from build123d import *

# Parameters (mm, degrees)
F0_W     = 60
F0_H     = 60
F0_R     = 1.25
F0_W_2   = 40.8
F0_H_2   = 40.8
F1_DEPTH = 7
F0_W_3   = 35
F0_H_3   = 35
F2_DEPTH = 2
F3_SIZE  = 1
F4_SIZE  = 1


with BuildPart() as f1:
    # F0 (on Front) → F1 (new body)
    with BuildSketch(Plane.XZ):
        Rectangle(F0_W, F0_H)
        with Locations((-25, -25)):
            Circle(F0_R, mode=Mode.SUBTRACT)
        with Locations((25, -25)):
            Circle(F0_R, mode=Mode.SUBTRACT)
        with Locations((-25, 25)):
            Circle(F0_R, mode=Mode.SUBTRACT)
        Rectangle(F0_W_2, F0_H_2, mode=Mode.SUBTRACT)
        with Locations((25, 25)):
            Circle(F0_R, mode=Mode.SUBTRACT)
    extrude(amount=F1_DEPTH)

    # F0 (on Front) → F2 (join)
    with BuildSketch(Plane.XZ):
        Rectangle(F0_W_2, F0_H_2)
        Rectangle(F0_W_3, F0_H_3, mode=Mode.SUBTRACT)
    extrude(amount=F2_DEPTH)

    # F3
    f3_edges = [f1.edges().sort_by_distance(p)[0] for p in [
        (20.4, -7, 0),
        (0, -7, 20.4),
        (-20.4, -7, 0),
        (0, -7, -20.4),
    ]]
    chamfer(f3_edges, length=F3_SIZE)

    # F4
    f4_edges = [f1.edges().sort_by_distance(p)[0] for p in [
        (-30, 0, 0),
        (0, 0, -30),
        (30, 0, 0),
        (0, 0, 30),
    ]]
    chamfer(f4_edges, length=F4_SIZE)


solid = f1.part
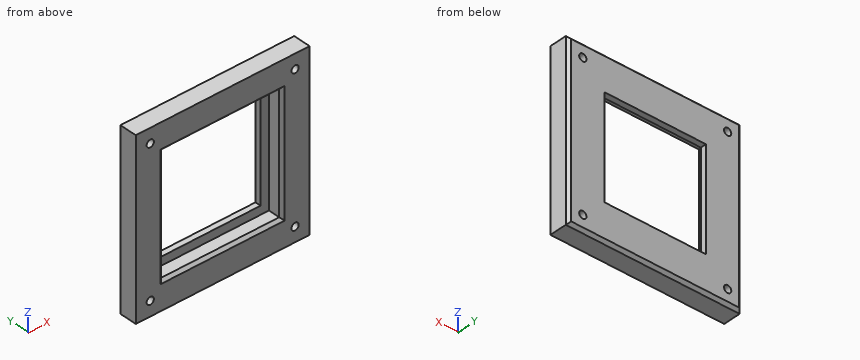
Check sheet for the modelled part. Datum: model origin and axes. Units: mm. Coordinates: 2 decimals unless noted, no trailing zeros. Loops run counter-clockwise (first coordinate to the right, second up) from the corner with the lowest first, then second, coordinate; pieces in that order, holes last. Notation, with made-up numbers: (45.5, 30.25) -> (75.5, 30.25) arc R18 ccw to (75.5, 55.25) -> close; hole circle Ø1 at (54, 86.25). An arc over 180 degrees is marked (long way). Write item = value, one per line. Start each with the question number.
1. Material ranges on line 1 (X direction, y = -5, z = 3.5); line 2 (Z direction, x = 25.5, y = -4.75), recorded low to high.
2. Section check D-D on y = -5. Record the cut outline in (x, z).
3. Section check C-C on x = -9.5. Record the cut outline in (y, z), then the cut area to 3 significant figures.
4. Depth check by flat-ended pin: P1, Ø5, axis at x = 3.5, z = -21.5, coming from the +Y side; P2, Ø1.5, axis at x = -25, z = -25, coming from the -Y side. Enter the tip coordinate at first touch or a pass-through.
5. Section check B-B on z = 14.5. Record the cut outline in (x, y), then the cut area to 3 significant figures.
6. Section check A-A on x = 25. Record the cut outline in (y, z).
Responses:
q1.line_1 = -30 to -20.4, 20.4 to 30
q1.line_2 = -30 to -26.15, -23.85 to 23.85, 26.15 to 30
q2.outline = (-30, -30) -> (30, -30) -> (30, 30) -> (-30, 30) -> close; hole circle Ø2.5 at (-25, -25); hole circle Ø2.5 at (-25, 25); hole (-20.4, -20.4) -> (20.4, -20.4) -> (20.4, 20.4) -> (-20.4, 20.4) -> close; hole circle Ø2.5 at (25, -25); hole circle Ø2.5 at (25, 25)
q3.outline = (-7, -30) -> (-1, -30) -> (0, -29) -> (0, -17.5) -> (-2, -17.5) -> (-2, -20.4) -> (-6, -20.4) -> (-7, -21.4) -> close; (-7, 21.4) -> (-6, 20.4) -> (-2, 20.4) -> (-2, 17.5) -> (0, 17.5) -> (0, 29) -> (-1, 30) -> (-7, 30) -> close
q3.area = 144 mm2
q4.P1 = 0
q4.P2 = through
q5.outline = (-30, -7) -> (-21.4, -7) -> (-20.4, -6) -> (-20.4, -2) -> (-17.5, -2) -> (-17.5, 0) -> (-29, 0) -> (-30, -1) -> close; (17.5, -2) -> (20.4, -2) -> (20.4, -6) -> (21.4, -7) -> (30, -7) -> (30, -1) -> (29, 0) -> (17.5, 0) -> close
q5.area = 144 mm2
q6.outline = (-7, -30) -> (-1, -30) -> (0, -29) -> (0, -26.25) -> (-7, -26.25) -> close; (-7, -23.75) -> (0, -23.75) -> (0, 23.75) -> (-7, 23.75) -> close; (-7, 26.25) -> (0, 26.25) -> (0, 29) -> (-1, 30) -> (-7, 30) -> close
